Read the model definition and answer for the solid it produces. Units are mm, in the model's axes. A direction names the side the tool comes from. Round coordinates to 2 decimals unless told otherwise and drop trailing zeros. Order: outer loops, then holes, each group sorted by start corner. A loop starts at its lowest first (then second) coordinate and runs counter-clockwise, first axis right, second up. Notation, with made-up numbers: (27, -24.75) -> (51, -24.75) arc R11 ccw to (51, -18.75) -> close; hole circle Ø5 at (37.25, 49). An arc over 180 degrees is marked (long way). Use a Markdown table: item, result. Add a question column.
1. Section B-B, the plane z = 0 is taken. Give the vertices of the cut face in (x, y).
2. Consider L1, parallel to Z at x = -3.25, y = 1.95; L2, parallel to Z at x = 1, y = 1.85; L3, parallel to X at y = 1.05, z = -3. Determine where each line is inside the solid, lowest interval first. Write a range as [from, to].
3. The mould has two halves that part along X. Classify faces 3 (the face through (2.454, 1.014, 0.082)), 4 (the face through (0, 1, 1.5)), 5 (the face through (0, 0, 2)), 6 (the face through (-1.08, 0.25, 4.88)): +X half, -X half, draft (parallel to the pull), parting line (faces both ways), or undercut.
4. Section D-D, the plane z = -1 is taken. Give the number of separate pieces and of enclosed holes in the cut face, then the cut area to 3 significant figures.
5. Section C-C, the plane y = 0.2 is taken. Give the vertices of the cut face in (x, z), then the cut area to 3 significant figures.
6. Given pin 1 (3 mm diameter, centred on x = -0.13, z = 3.45, fed in from -Y), flat-ended and moving along its own axis, determine where the tip first touches the part or whether it passes through.
7. For faces 1 (the face through (1.5, 1, 0)), 2 (the face through (0, 2, 2)), determine the directions among +Z, -Z, +X, -X, +Y, -Y from which every point of the face is accessible in a straight line to the end or side of a thin tool.
8. Section A-A, the plane x = 0 is taken. Give the vertices of the cut face in (y, z).
```python
from build123d import *

# Parameters (mm, degrees)
SKIZZE1_R                       = 5
AUFSATZ_LINEAR_AUSTRAGEN1_DEPTH = 2
SKIZZE3_W                       = 3
SKIZZE3_H                       = 3
SCHNITT_LINEAR_AUSTRAGEN1_DEPTH = 3
SKIZZE4_R                       = 1
SCHNITT_LINEAR_AUSTRAGEN2_DEPTH = 3
KREISMUSTER1_COUNT              = 4


with BuildPart() as part:
    # Skizze1 → Aufsatz-Linear austragen1 (new body)
    with BuildSketch(Plane(origin=(0, 0, 0), x_dir=(1, 0, 0), z_dir=(0, 1, 0))):
        Circle(SKIZZE1_R)
    extrude(amount=AUFSATZ_LINEAR_AUSTRAGEN1_DEPTH)

    # Skizze3 → Schnitt-Linear austragen1 (cut)
    with BuildSketch(Plane(origin=(0, 2, 0), x_dir=(1, 0, 0), z_dir=(0, 1, 0))):
        Rectangle(SKIZZE3_W, SKIZZE3_H)
    extrude(amount=-SCHNITT_LINEAR_AUSTRAGEN1_DEPTH, mode=Mode.SUBTRACT)

    # Skizze4 → Schnitt-Linear austragen2 (cut)
    with BuildSketch(Plane(origin=(0, 2, 0), x_dir=(1, 0, 0), z_dir=(0, 1, 0))):
        with Locations((3.452809927, -0.126446108)):
            Circle(SKIZZE4_R)
    schnitt_linear_austragen2 = extrude(amount=-SCHNITT_LINEAR_AUSTRAGEN2_DEPTH, mode=Mode.SUBTRACT)

    # Kreismuster1: Schnitt-Linear austragen2 ×4 about axis
    kreismuster1_axis = Axis((0, 0, 0), (0, 1, 0))
    for i in range(1, KREISMUSTER1_COUNT):
        add(schnitt_linear_austragen2.rotate(kreismuster1_axis, i * 360 / KREISMUSTER1_COUNT), mode=Mode.SUBTRACT)

    # Skizze6 → Schnitt-Rotation2 (revolve, cut)
    with BuildSketch(Plane.XY):
        with BuildLine():
            Line((-5, 1.5), (-5, 0.5))
            ThreePointArc((-5, 0.5), (-4.5, 1), (-5, 1.5))
        make_face()
    revolve(axis=Axis((0, 2, 0), (0, -1, 0)), mode=Mode.SUBTRACT)


solid = part.part
```
Verdict:
| question | item | result |
|---|---|---|
| 1 | outline | (-5, 0) -> (-4.44, 0) -> (-4.44, 2) -> (-5, 2) -> (-5, 1.5) arc R0.5 cw to (-5, 0.5) -> close; (-2.46, 0) -> (-1.5, 0) -> (-1.5, 2) -> (-2.46, 2) -> close; (1.5, 0) -> (2.46, 0) -> (2.46, 2) -> (1.5, 2) -> close; (4.44, 0) -> (5, 0) -> (5, 0.5) arc R0.5 cw to (5, 1.5) -> (5, 2) -> (4.44, 2) -> close |
| 2 | L1 | z = [-3.8, -1.11], [0.85, 3.8] |
| 2 | L2 | z = [-4.9, -3.94], [-2.97, -1.5], [1.5, 4.9] |
| 2 | L3 | x = [-3.36, -0.77], [1.02, 3.36] |
| 3 | face 3 | undercut |
| 3 | face 4 | undercut |
| 3 | face 5 | draft |
| 3 | face 6 | parting line |
| 4 | separate pieces | 3 |
| 4 | enclosed holes | 0 |
| 4 | area | 10.8 mm2 |
| 5 | outline | circle Ø10 at (0, 0); hole circle Ø2 at (-3.45, -0.13); hole (-1.5, -1.5) -> (1.5, -1.5) -> (1.5, 1.5) -> (-1.5, 1.5) -> close; hole circle Ø2 at (-0.13, 3.45); hole circle Ø2 at (0.13, -3.45); hole circle Ø2 at (3.45, 0.13) |
| 5 | area | 57.0 mm2 |
| 6 | pin 1 | stops at y = 0 |
| 7 | face 1 | +Y, -Y |
| 7 | face 2 | +Z, -Z, +X, -X, +Y |
| 8 | outline | (0, -5) -> (0.5, -5) arc R0.5 cw to (1.5, -5) -> (2, -5) -> (2, -4.44) -> (0, -4.44) -> close; (0, -2.46) -> (2, -2.46) -> (2, -1.5) -> (0, -1.5) -> close; (0, 1.5) -> (2, 1.5) -> (2, 2.46) -> (0, 2.46) -> close; (0, 4.44) -> (2, 4.44) -> (2, 5) -> (1.5, 5) arc R0.5 cw to (0.5, 5) -> (0, 5) -> close |
